from build123d import *

# Parameters (mm, degrees)
F0_R     = 4.445
F1_DEPTH = 13.97
F2_R     = 9.525
F2_R_2   = 6.985
F3_DEPTH = 7.874
F5_DEPTH = 4.572
F6_R     = 0.762
F7_DEPTH = 5.08


with BuildPart() as f1:
    # F0 (on Top) → F1 (new body)
    with BuildSketch(Plane.XY):
        Polygon((11.0871, -6.4011401695), (11.0871, 6.4011401695), (0, 12.8022803391), (-11.0871, 6.4011401695), (-11.0871, -6.4011401695), (0, -12.8022803391), align=None)
        Circle(F0_R, mode=Mode.SUBTRACT)
    extrude(amount=F1_DEPTH)

    # F2 (on face) → F3 (cut)
    with BuildSketch(Plane(origin=(0, 0, 0), x_dir=(1, 0, 0), z_dir=(0, 0, -1))):
        Circle(F2_R)
        Circle(F2_R_2, mode=Mode.SUBTRACT)
    extrude(amount=-F3_DEPTH, mode=Mode.SUBTRACT)

    # F4 (on face) → F5 (cut)
    with BuildSketch(Plane.XY.offset(13.97)):
        Polygon((-6.35, 3.6661742094), (-6.35, -3.6661742094), (0, -7.3323484187), (6.35, -3.6661742094), (6.35, 3.6661742094), (0, 7.3323484187), align=None)
    extrude(amount=-F5_DEPTH, mode=Mode.SUBTRACT)

    # F6
    f6_edges = [f1.edges().sort_by_distance(p)[0] for p in [
        (-9.525, 0, 7.874),
        (-6.985, 0, 7.874),
    ]]
    fillet(f6_edges, radius=F6_R)

    # F7 (cut): a face of the model
    f7_faces = [f1.faces().sort_by_distance(p)[0] for p in [
        (-6.7874343653, 0, 0),
    ]]
    extrude(f7_faces, amount=-F7_DEPTH, mode=Mode.SUBTRACT)


solid = f1.part
The model under review builds one solid part; all positions refer to its coordinate system, in mm. A direction names the side the tool comes from. Round coordinates to 2 decimals unless told otherwise and drop trailing zeros. Order: outer loops, then holes, each group sorted by start corner. A loop starts at its lowest first (then second) coordinate and runs counter-clockwise, first axis right, second up. Notation, with made-up numbers: (26, -39.75) - (78, -39.75) arc R19 cw to (78, -28.75) - close; hole circle Ø2 at (-3, 69). An arc over 180 degrees is marked (long way). Use one line per item in the form item = value.
Q1. Add section B-B on y = 0. Give the boundary of the cut face in (x, z) (3 decimals), then the cut area to 3 significant figures.
Response values:
outline = (-11.087, 0) - (-9.525, 0) - (-9.525, 7.112) arc R0.762 cw to (-8.763, 7.874) - (-7.747, 7.874) arc R0.762 cw to (-6.985, 7.112) - (-6.985, 5.08) - (-4.445, 5.08) - (-4.445, 9.398) - (-6.35, 9.398) - (-6.35, 13.97) - (-11.087, 13.97) - close; (4.445, 5.08) - (6.985, 5.08) - (6.985, 7.112) arc R0.762 cw to (7.747, 7.874) - (8.763, 7.874) arc R0.762 cw to (9.525, 7.112) - (9.525, 0) - (11.087, 0) - (11.087, 13.97) - (6.35, 13.97) - (6.35, 9.398) - (4.445, 9.398) - close
area = 103 mm^2
Q2. Add section A-A on z = 6. Give the boundary of the cut face in (x, y) (3 decimals).
Response values:
outline = (-11.087, -6.401) - (0, -12.802) - (11.087, -6.401) - (11.087, 6.401) - (0, 12.802) - (-11.087, 6.401) - close; circle Ø13.97 at (0, 0); hole circle Ø19.05 at (0, 0); hole circle Ø8.89 at (0, 0)
Q3. Clearance check with flat-ended pins moving along their axes: P1, Ø4, axis at y = -9.5, z = 11.5, coming from the -X side; P2, Ø8, axis at x = 7.5, y = 6.5, coming from the -Z side; P3, Ø7, axis at x = 0, y = 3.5, coming from the -Z side; P4, Ø11.5, axis at x = 0, y = 0, coming from the +Z side. State where each tip first meets the part, or that it passes through.
Response values:
P1 = -9.18
P2 = 0
P3 = 5.08
P4 = 9.4
Q4. Mouldability with a two-part tool opening along X and no side actions: class faces 4 (the flat face through (3.131, -5.525, 11.716)), 5 (the flat face through (-5, -8.5, 0)), 6 (the flat face through (-11.087, 0, 7)), 7 (the flat face through (5.621, 9.557, 6.887)) as pulls with the +X half, pulls with the -X half, needs draft (parallel to the pull), parting line crosses it, or undercut.
Response values:
face_4 = undercut
face_5 = needs draft
face_6 = pulls with the -X half
face_7 = pulls with the +X half
Q5. To check wall thickness, follow line 1 (X direction, y = 0, z = 4.5) (3 decimals); line 2 (X direction, y = 0, z = 7.95) (3 decimals); line 3 (X direction, y = 0, z = 5.5) (3 decimals). State the ranges of each line that lie inside material, in increasing order.
Response values:
line_1 = -11.087 to -9.525, 9.525 to 11.087
line_2 = -11.087 to -4.445, 4.445 to 11.087
line_3 = -11.087 to -9.525, -6.985 to -4.445, 4.445 to 6.985, 9.525 to 11.087
Q6. Tool access review of faces 1 (the flat face through (6.35, 0, 12)), 2 (the flat face through (-5, -6, 13.97)), 3 (the flat face through (0, -5, 5.08)): name each direction out of +Z, -Z, +X, -X, +Y, -Y from which nothing blocks a thin tool from reaching the whole face with its end or side.
Response values:
face_1 = +Z
face_2 = +Z, +X, -X, +Y, -Y
face_3 = -Z
Q7. Add section C-C on z = 10.5. Give the boundary of the cut face in (x, y).
Response values:
outline = (-11.09, -6.4) - (0, -12.8) - (11.09, -6.4) - (11.09, 6.4) - (0, 12.8) - (-11.09, 6.4) - close; hole (-6.35, -3.67) - (0, -7.33) - (6.35, -3.67) - (6.35, 3.67) - (0, 7.33) - (-6.35, 3.67) - close
Q8. Add section D-D on z = 4.5. Give the boundary of the cut face in (x, y) (3 decimals), then the cut area to 3 significant figures.
Response values:
outline = (-11.087, -6.401) - (0, -12.802) - (11.087, -6.401) - (11.087, 6.401) - (0, 12.802) - (-11.087, 6.401) - close; hole circle Ø19.05 at (0, 0)
area = 141 mm^2
